```python
from build123d import *

# Parameters (mm, degrees)
SKETCH1_W               = 180
SKETCH1_H               = 60
BOSS_EXTRUDE1_DEPTH     = 3.175
SKETCH5_W               = 20.1
SKETCH5_H               = 20.1
CUT_EXTRUDE1_DEPTH      = 1
CUT_EXTRUDE1_DEPTH_BACK = 4.175
M4_CLEARANCE_HOLE2_D    = 4.5
FILLET2_R               = 4


with BuildPart() as part:
    # Sketch1 → Boss-Extrude1 (new body)
    with BuildSketch(Plane(origin=(0, 0, 0), x_dir=(1, 0, 0), z_dir=(0, 1, 0))):
        Rectangle(SKETCH1_W, SKETCH1_H)
    extrude(amount=BOSS_EXTRUDE1_DEPTH)

    # Sketch5 → Cut-Extrude1 (cut, two sides)
    with BuildSketch(Plane(origin=(0, 3.175, 0), x_dir=(1, 0, 0), z_dir=(0, 1, 0))) as cut_extrude1_sk:
        with Locations((79.95, 19.95)):
            Rectangle(SKETCH5_W, SKETCH5_H)
    extrude(amount=CUT_EXTRUDE1_DEPTH, mode=Mode.SUBTRACT)
    extrude(cut_extrude1_sk.sketch, amount=-CUT_EXTRUDE1_DEPTH_BACK, mode=Mode.SUBTRACT)

    # M4 Clearance Hole2 (through all)
    with Locations(Plane(origin=(0, 3.175, 0), x_dir=(1, 0, 0), z_dir=(0, 1, 0))):
        with Locations((-70, 20), (40, 20), (80, -20)):
            Hole(M4_CLEARANCE_HOLE2_D / 2)

    # Fillet2
    fillet2_edges = [part.edges().sort_by_distance(p)[0] for p in [
        (69.9, 1.5875, -9.9),
        (69.9, 1.5875, -30),
        (90, 1.5875, -9.9),
        (-90, 1.5875, -30),
        (90, 1.5875, 30),
        (-90, 1.5875, 30),
    ]]
    fillet(fillet2_edges, radius=FILLET2_R)


solid = part.part
```
Can you work these out from the model? Positions are in its coordinate system, mm. A direction names the side the tool comes from. Give positions to 0.01 mm unless a question says otherwise; leave off trailing zeros. Loops run counter-clockwise (first coordinate to the right, second up) from the corner with the lowest first, then second, coordinate; pieces in that order, holes last. Notation, with made-up numbers: M -34.5,-6.5 L -8.5,-6.5 A20 ccw -8.5,10.5 Z; hole C 51.5,-39 d3. An arc over 180 degrees is marked long. Answer in a Markdown table with one row per item.
1. Which directions (+Z, -Z, +X, -X, +Y, -Y) give clear straight access to the entire face, cutting with the end or side of a thin tool? Please do faces 1 (the flat face through (-1, 0, 0)), 2 (the flat face through (80, 2, -9.9)).
Taken from the geometry:
| item | result |
|---|---|
| face 1 | +Z, -Z, +X, -X, -Y |
| face 2 | -Z, +X, +Y, -Y |
2. Suppose I cut it at B-B on y = 1.55. Write out the boundary of the cut face in (x, z).
Taken from the geometry:
| item | result |
|---|---|
| outline | M -90,-26 A4 ccw -86,-30 L 65.9,-30 A4 ccw 69.9,-26 L 69.9,-13.9 A4 cw 73.9,-9.9 L 86,-9.9 A4 ccw 90,-5.9 L 90,26 A4 ccw 86,30 L -86,30 A4 ccw -90,26 Z; hole C -70,-20 d4.5; hole C 40,-20 d4.5; hole C 80,20 d4.5 |
3. If I drill on line 1 along X through (y, z) = (1.15, -20); line 2 along Z through (x, y) = (80, 1.85); line 3 along Z through (x, y) = (40, 1.6), over which ranges is the centre line in solid material (lowest first)?
Taken from the geometry:
| item | result |
|---|---|
| line 1 | x = -90 to -72.25, -67.75 to 37.75, 42.25 to 69.9 |
| line 2 | z = -9.9 to 17.75, 22.25 to 30 |
| line 3 | z = -30 to -22.25, -17.75 to 30 |
4. Suppose I cut it at C-C on x = -70. Write out the boundary of the cut face in (y, z) (3 decimals), plus the area to 3 significant figures.
Taken from the geometry:
| item | result |
|---|---|
| outline | M 0,-30 L 3.175,-30 L 3.175,-22.25 L 0,-22.25 Z; M 0,-17.75 L 3.175,-17.75 L 3.175,30 L 0,30 Z |
| area | 176 mm² |
5. For pin 1 Ø12 at (x, z) = (18, 3.5) entering from -Y, with a flat end and sliding along its axis, tell me the tip position at first contact or that it passes through.
Taken from the geometry:
| item | result |
|---|---|
| pin 1 | stops at y = 0 |
6. Thinking about a two-plate mould opening in Z: for faces 3 (the cylindrical face through (40.488, 1.565, -17.804)), 4 (the cylindrical face through (77.92, 1.57, 20.86)), 5 (the cylindrical face through (88.797, 1.61, 28.859)), 6 (the flat face through (90, 2, 10)), which applies, released by +Z, released by -Z, zero draft, split by the parting line, or undercut?
Taken from the geometry:
| item | result |
|---|---|
| face 3 | undercut |
| face 4 | undercut |
| face 5 | released by +Z |
| face 6 | zero draft |
7. Suppose I cut it at A-A on z = 20. Write out the boundary of the cut face in (x, y) (3 decimals).
Taken from the geometry:
| item | result |
|---|---|
| outline | M -90,0 L 77.75,0 L 77.75,3.175 L -90,3.175 Z; M 82.25,0 L 90,0 L 90,3.175 L 82.25,3.175 Z |
